Geometry check sheet. Reference: drawing and pictorial views, mm from the part's lowest x, y, z. A direction names the side the tool comes from. Round coordinates to 2 decimals unless told otherwise and drop trailing zeros. Write each loop counter-clockwise with the first axis right and the second up, starting at its lowest first coordinate (ties: lowest second). Pieces come first, ordered by that corner, then holes.
Item 1: Section check D-D, the plane z = 5.25. Record the cut outline in (x, y), plus the area to 3 significant figures.
Item 2: Section check C-C, the plane y = 10. Record the cut outline in (x, z), plus the area to 3 significant figures.
Item 3: Depth check by flat-ended pin: pin 1 (1.5 mm diameter, centred on y = 13, z = 1.5, fed in from +X); pin 2 (2 mm diameter, centred on y = 4.5, z = 1.5, fed in from -X). Enter the tip coordinate at first touch or a pass-through.
Item 4: Section check A-A, the plane x = 10. Record the cut outline in (y, z).
Item 5: Section check B-B, the plane y = 13. Record the cut outline in (x, z), plus the area to 3 significant figures.
Item 6: Release check for a two-part mould opening along Y. For the marked faces 1, 2 and 3 record: pulls with the +Y half, pulls with the -Y half, needs draft (parallel to the pull), parting line crosses it, or undercut.
Item 7: Set-up check for the marked faces 4 and 5: record each of +Z, -Z, +X, -X, +Y, -Y from which the full face is reachable in a straight line by a thin tool's end or side.
Item 8: Material ranges on line 1 along Y through (x, z) = (10, 2); line 2 along Y through (x, z) = (10, 5.5); line 3 along X through (y, z) = (7, 5.75), recorded low to high.
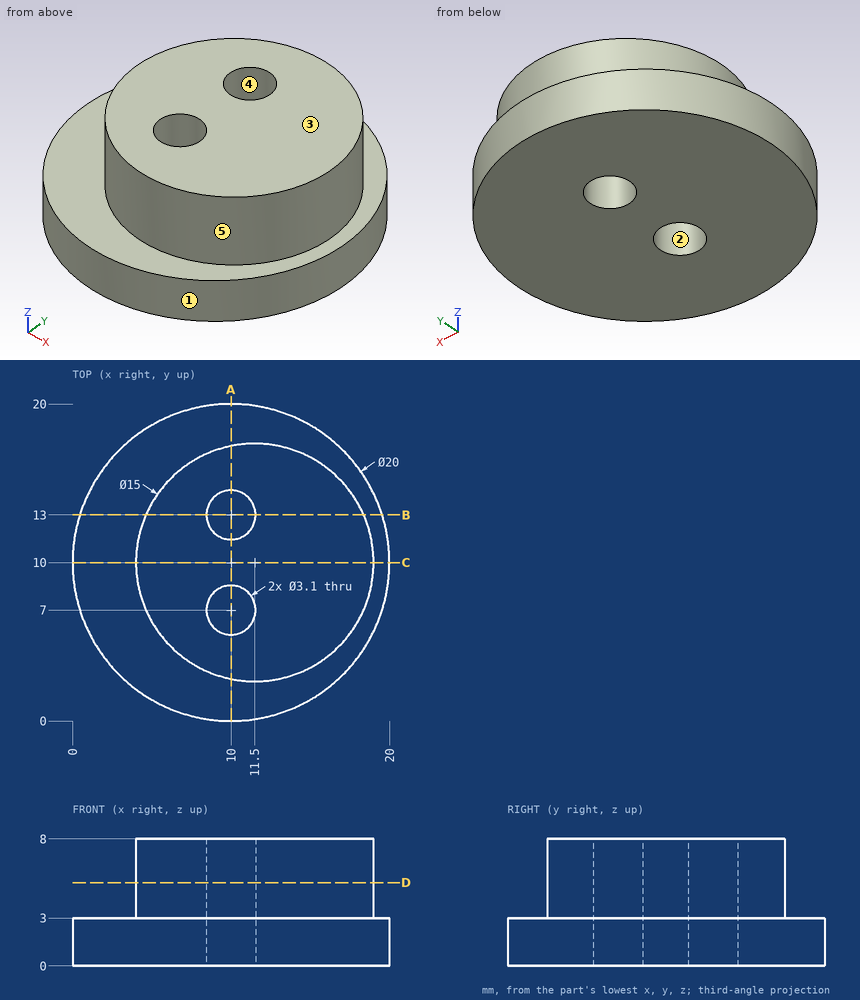
Values found:
1. outline: circle Ø15 at (11.5, 10); hole circle Ø3.1 at (10, 7); hole circle Ø3.1 at (10, 13)
1. area: 162 mm2
2. outline: (0, 0) - (20, 0) - (20, 3) - (19, 3) - (19, 8) - (4, 8) - (4, 3) - (0, 3) - close
2. area: 135 mm2
3. pin 1: stops at x = 19.74
3. pin 2: stops at x = 1.07
4. outline: (0, 0) - (5.45, 0) - (5.45, 8) - (2.65, 8) - (2.65, 3) - (0, 3) - close; (8.55, 0) - (11.45, 0) - (11.45, 8) - (8.55, 8) - close; (14.55, 0) - (20, 0) - (20, 3) - (17.35, 3) - (17.35, 8) - (14.55, 8) - close
5. outline: (0.46, 0) - (8.45, 0) - (8.45, 8) - (4.63, 8) - (4.63, 3) - (0.46, 3) - close; (11.55, 0) - (19.54, 0) - (19.54, 3) - (18.37, 3) - (18.37, 8) - (11.55, 8) - close
5. area: 101 mm2
6. face 1: parting line crosses it
6. face 2: undercut
6. face 3: needs draft
7. face 4: +Z, -Z
7. face 5: +Z
8. line 1: y = 0 to 5.45, 8.55 to 11.45, 14.55 to 20
8. line 2: y = 2.65 to 5.45, 8.55 to 11.45, 14.55 to 17.35
8. line 3: x = 4.63 to 8.45, 11.55 to 18.37
